Check sheet for the drawn part. Datum: minimum x, y, z corner. Units: mm. Coordinates: 2 decimals unless noted, no trailing zeros. Write each loop counter-clockwise with the first axis right and the second up, starting at its lowest first coordinate (ties: lowest second). Pieces come first, ordered by that corner, then holes. Notation, with made-up numbers: M 47.5,-39 L 106.5,-39 A25 cw 106.5,-16 Z; hole C 54.25,66 d4. An arc over 180 degrees is marked long. Answer in a Markdown table with one row per item.
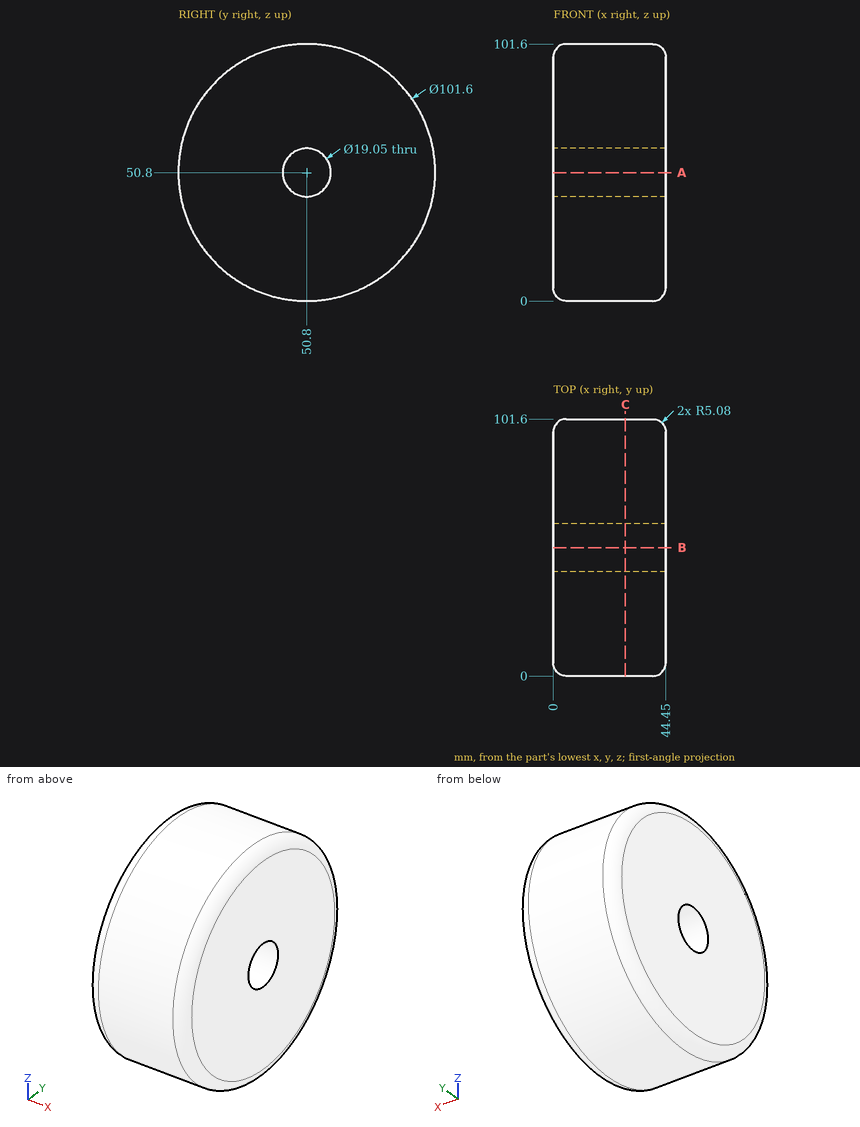
1) Depth check by flat-ended pin: pin 1 (1 mm diameter, centred on x = 21.5, z = 32.5, fed in from -Y); pin 2 (1.5 mm diameter, centred on x = 28, y = 68.5, fed in from -Z); pin 3 (10 mm diameter, centred on x = 24, y = 23, fed in from -Z); pin 4 (10 mm diameter, centred on y = 51, z = 41.5, fed in from +X). Enter the tip coordinate at first touch or a pass-through.
Response values:
| item | result |
|---|---|
| pin 1 | stops at y = 3.22 |
| pin 2 | stops at z = 2.91 |
| pin 3 | stops at z = 5.4 |
| pin 4 | stops at x = 44.45 |
2) Sectioned sample at A-A (z = 50.8). Record the cut outline in (x, y) (3 decimals), then the cut area to 3 significant figures.
Response values:
| item | result |
|---|---|
| outline | M 0,5.08 A5.08 ccw 5.08,0 L 39.37,0 A5.08 ccw 44.45,5.08 L 44.45,41.275 L 0,41.275 Z; M 0,60.325 L 44.45,60.325 L 44.45,96.52 A5.08 ccw 39.37,101.6 L 5.08,101.6 A5.08 ccw 0,96.52 Z |
| area | 3,650 mm² |
3) Sectioned sample at C-C (x = 28.5). Record the cut outline in (y, z) (3 decimals).
Response values:
| item | result |
|---|---|
| outline | C 50.8,50.8 d101.6; hole C 50.8,50.8 d19.05 |
4) Thickness scan on L1, parallel to Z at x = 17.5, y = 50.8 (3 decimals); L2, parallel to Y at x = 27, z = 57; L3, parallel to Z at x = 6, y = 49.5. Record the ranges inside material, lowest first. Write a range as [from, to].
Response values:
| item | result |
|---|---|
| L1 | z = [0, 41.275], [60.325, 101.6] |
| L2 | y = [0.38, 43.57], [58.03, 101.22] |
| L3 | z = [0.02, 41.36], [60.24, 101.58] |
